```python
from build123d import *

# Parameters (mm, degrees)
ESQUISSE1_W             = 300
ESQUISSE1_H             = 95
BOSS_EXTRU_1_DEPTH      = 5
BOSS_EXTRU_2_DEPTH      = 300
BOSS_EXTRU_3_DEPTH      = 10
ESQUISSE6_R             = 5
ENL_V_MAT_EXTRU_2_DEPTH = 16
ESQUISSE7_W             = 290
ESQUISSE7_H             = 23.020862504
ENL_V_MAT_EXTRU_3_DEPTH = 30


with BuildPart() as part:
    # Esquisse1 → Boss.-Extru.1 (new body)
    with BuildSketch(Plane.XY):
        with Locations((150, 47.5)):
            Rectangle(ESQUISSE1_W, ESQUISSE1_H)
    extrude(amount=BOSS_EXTRU_1_DEPTH)

    # Esquisse3 → Boss.-Extru.2 (add)
    with BuildSketch(Plane.ZY):
        Polygon((-5, 0), (0, 0), (0, 5), align=None)
    extrude(amount=-BOSS_EXTRU_2_DEPTH)

    # Esquisse5 → Boss.-Extru.3 (add)
    with BuildSketch(Plane.XY.offset(5)):
        Polygon((195, 95), (105, 95), (0, 95), (0, 30), (0, 0), (300, 0), (300, 30), (300, 95), align=None)
    extrude(amount=BOSS_EXTRU_3_DEPTH)

    # Esquisse6 → Enlèv. mat.-Extru.2 (cut, through all)
    with BuildSketch(Plane(origin=(0, 0, 0), x_dir=(-1, 0, 0), z_dir=(0, 0, -1))):
        with Locations((-180, 75)):
            Circle(ESQUISSE6_R)
        with Locations((-180, 45)):
            Circle(ESQUISSE6_R)
        with Locations((-120, 45)):
            Circle(ESQUISSE6_R)
        with Locations((-120, 75)):
            Circle(ESQUISSE6_R)
    extrude(amount=-ENL_V_MAT_EXTRU_2_DEPTH, mode=Mode.SUBTRACT)

    # Esquisse7 → Enlèv. mat.-Extru.3 (cut)
    with BuildSketch(Plane.XZ):
        with Locations((150, 16.510431252)):
            Rectangle(ESQUISSE7_W, ESQUISSE7_H)
    extrude(amount=-ENL_V_MAT_EXTRU_3_DEPTH, mode=Mode.SUBTRACT)


solid = part.part
```
Geometry check sheet. Reference: the model listing, model coordinates, mm. A direction names the side the tool comes from. Round coordinates to 2 decimals unless told otherwise and drop trailing zeros. Order: outer loops, then holes, each group sorted by start corner. A loop starts at its lowest first (then second) coordinate and runs counter-clockwise, first axis right, second up. Notation, with made-up numbers: M 17.25,-33.5 L 49.25,-33.5 A16 ccw 49.25,-12.5 Z; hole C -39,6.5 d7. An arc over 180 degrees is marked long. Answer as CSV lines item,"result".
1) Mould release check, pull along X, two halves, no side actions. Record for faces 4 (the face through (0, 48, 7)), 5 (the face through (148, 15, 5)), 6 (the face through (152, 95, 7)): +X half, -X half, draft (parallel to the pull), parting line (faces both ways), or undercut.
Entries:
face 4,"-X half"
face 5,"undercut"
face 6,"draft"
2) Sectioned sample at B-B on y = 45. Record the cut outline in (x, z), and give its area (3 significant figures).
Entries:
outline,"M 0,0 L 115,0 L 115,15 L 0,15 Z; M 125,0 L 175,0 L 175,15 L 125,15 Z; M 185,0 L 300,0 L 300,15 L 185,15 Z"
area,"4,200 mm2"
3) Sectioned sample at A-A on x = 120. Record the cut outline in (y, z).
Entries:
outline,"M 0,-5 L 5,0 L 40,0 L 40,15 L 30,15 L 30,5 L 0,5 Z; M 50,0 L 70,0 L 70,15 L 50,15 Z; M 80,0 L 95,0 L 95,15 L 80,15 Z"
4) Sectioned sample at D-D on x = 68. Record the cut outline in (y, z).
Entries:
outline,"M 0,-5 L 5,0 L 95,0 L 95,15 L 30,15 L 30,5 L 0,5 Z"
5) Gauge pin test, flat ends, axial feed: pin 1 Ø12 at (x, z) = (102, 4) entering from -Y; pin 2 Ø13 at (x, y) = (120, 45) entering from -Z; pin 3 Ø15 at (x, y) = (218, 19) entering from +Z. Record the tip position at first contact, or that the pin passes through.
Entries:
pin 1,"y = 0"
pin 2,"z = 0"
pin 3,"z = 5"
6) Thickness scan on probe 1 along Y at (x, z) = (120, 12.25); probe 2 along X at (y, z) = (29.5, 10.75); probe 3 along Z at (x, y) = (76, 65.5). Record the ranges inside material, lowest first. Write a range as [from, to].
Entries:
probe 1,"[30, 40], [50, 70], [80, 95]"
probe 2,"[0, 5], [295, 300]"
probe 3,"[0, 15]"
7) Sectioned sample at C-C on y = 10. Record the cut outline in (x, z).
Entries:
outline,"M 0,0 L 300,0 L 300,15 L 295,15 L 295,5 L 5,5 L 5,15 L 0,15 Z"
8) Tool access check on faces 1 (the face through (148, 0, 0)), 2 (the face through (5, 15, 10)), 3 (the face through (148, 51, 0)). Record the directions out of +Z, -Z, +X, -X, +Y, -Y that give a thin tool (end or side, any length) a straight path to the whole face; none if there is none.
Entries:
face 1,"+Z, -Z, +X, -X, -Y"
face 2,"+Z, -Y"
face 3,"-Z, +X, -X, +Y"
